For this review, use the dimensioned drawing (mm, ordinates from the lowest corner) and the shaded views. A direction names the side the tool comes from. Give positions to 0.01 mm unless a question says otherwise; leave off trailing zeros. Write each loop counter-clockwise with the first axis right and the second up, starting at its lowest first coordinate (ties: lowest second). Pieces come first, ordered by that corner, then holes.
1) For P1, Ø1, axis at x = 34.5, z = 6.5, coming from the -Y side (1 decimal); P2, Ø3.5, axis at x = 4.5, z = 6.5, coming from the +Y side; P3, Ø4, axis at y = 12, z = 2, coming from the +X side, all flat-tipped, find the tip position at first contact; note any pin that passes through.
2) We need section B-B on z = 5.75. Give the number of separate pieces and of enclosed holes in the cut face.
3) We need section A-A on x = 5. Give the boundary of the cut face in (y, z), and give its area (3 significant figures).
4) Wall thickness on line 1 along Z through (x, y) = (5, 1.2); line 2 along Y through (x, z) = (7.5, 7.5); line 3 along X through (y, z) = (4, 8): over which ranges is each line inside the solid? List them lowest first.
5) We need section D-D on y = 2.5. Give the boundary of the cut face in (x, z).
6) We need section C-C on y = 9.5. Give the boundary of the cut face in (x, z).
7) Machinability: for the marked faces 1, 2 and 3, which of the approach directions +Z, -Z, +X, -X, +Y, -Y give a long, thin tool a straight path to every point of the face, cutting with its end or side? Answer none if there is none.
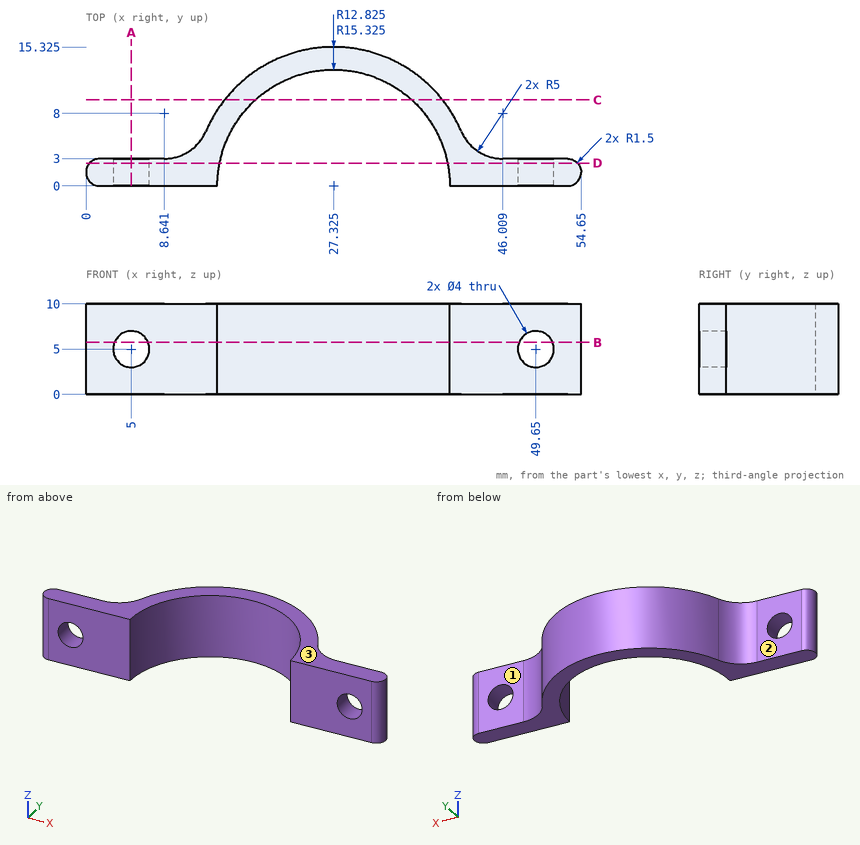
Results list:
1. P1: stops at y = 10.3
1. P2: stops at y = 3
1. P3: stops at x = 38.94
2. separate pieces: 3
2. enclosed holes: 0
3. outline: (0, 0) - (3, 0) - (3, 3) - (0, 3) - close; (0, 7) - (3, 7) - (3, 10) - (0, 10) - close
3. area: 18.0 mm2
4. line 1: z = 0 to 3, 7 to 10
4. line 2: y = 0 to 3
4. line 3: x = 11.64 to 15.14, 39.51 to 43.01
5. outline: (0.38, 0) - (14.75, 0) - (14.75, 10) - (0.38, 10) - close; (39.9, 0) - (54.27, 0) - (54.27, 10) - (39.9, 10) - close; hole circle Ø4 at (5, 5); hole circle Ø4 at (49.65, 5)
6. outline: (15.3, 0) - (18.71, 0) - (18.71, 10) - (15.3, 10) - close; (35.94, 0) - (39.35, 0) - (39.35, 10) - (35.94, 10) - close
7. face 1: +Z, -Z, +X, +Y
7. face 2: +Z, -Z, -X, +Y
7. face 3: +Z, +X, -X, +Y, -Y
